```python
from build123d import *

# Parameters (mm, degrees)
BOSS_EXTRUDE1_DEPTH    = 558.8
SKETCH2_W              = 1233.22752028
SKETCH2_H              = 1270
SKETCH2_W_2            = 864.480609306
SKETCH2_H_2            = 355.6
CUT_EXTRUDE1_DEPTH     = 756.196292364
FILLET1_R              = 213.36
FILLET2_R              = 76.2
FILLET5_R              = 106.68
SHELL1_T               = 19.05
SKETCH7_W              = 20.32
SKETCH7_H              = 152.4
SKETCH7_2_W            = 20.32
SKETCH7_2_H            = 152.4
CUT_EXTRUDE2_DEPTH     = 152.4
FILLET6_R              = 25.4
LPATTERN1_COUNT        = 3
LPATTERN1_PITCH        = 167.64
FILLET6_OF_LPATTERN1_R = 25.4
SKETCH10_R             = 12.7
CUT_EXTRUDE3_DEPTH     = 688.251792528


with BuildPart() as part:
    # Sketch1 → Boss-Extrude1 (new body)
    with BuildSketch(Plane(origin=(0, 0, 0), x_dir=(1, 0, 0), z_dir=(0, 1, 0))):
        Polygon((359.210244843, 0), (0, -359.210244843), (-359.210244843, 0), (0, 359.210244843), align=None)
    extrude(amount=BOSS_EXTRUDE1_DEPTH)

    # Sketch2 → Cut-Extrude1 (cut, through all)
    with BuildSketch(Plane(origin=(0, 558.8, 0), x_dir=(1, 0, 0), z_dir=(0, 1, 0))):
        with Locations((0, 127)):
            Rectangle(SKETCH2_W, SKETCH2_H)
        with Locations((0, 127)):
            Rectangle(SKETCH2_W_2, SKETCH2_H_2, mode=Mode.SUBTRACT)
    extrude(amount=-CUT_EXTRUDE1_DEPTH, mode=Mode.SUBTRACT)

    # Fillet1
    # the kernel refuses this fillet: 213.36 mm, written as the material it takes off along each edge
    with BuildSketch(Plane(origin=(359.210244843, -399.180090434, 0), x_dir=(-0.707106781186546, 0, 0.707106781186549), z_dir=(0, 1, 0))) as fillet1_piece_1:
        with BuildLine():
            CenterArc((213.36, -159.672036174), FILLET1_R, 131.550696865, 48.449303135)
            Line((0, -159.672036174), (-4.2672, -159.672036174))
            Line((-4.2672, -159.672036174), (-4.2672, 0))
            Line((-4.2672, 0), (0, 4.2672))
            ThreePointArc((0, 4.2672), (35.921024484, 4.2672), (69.011689948, 3.193440723))
            Line((69.011689948, 3.193440723), (71.842048969, 0))
        make_face()
    extrude(amount=1357.160180869, mode=Mode.SUBTRACT)
    with BuildSketch(Plane(origin=(-359.210244843, -399.180090434, 0), x_dir=(0.707106781186546, 0, -0.7071067811865489), z_dir=(0, 1, 0))) as fillet1_piece_2:
        with BuildLine():
            CenterArc((159.672036174, -213.36), FILLET1_R, 90, 48.449303135)
            Line((0, -71.842048969), (-3.193440723, -69.011689948))
            ThreePointArc((-3.193440723, -69.011689948), (-4.2672, -35.921024484), (-4.2672, 0))
            Line((-4.2672, 0), (0, 4.2672))
            Line((0, 4.2672), (159.672036174, 4.2672))
            Line((159.672036174, 4.2672), (159.672036174, 0))
        make_face()
    extrude(amount=1357.160180869, mode=Mode.SUBTRACT)

    # Fillet2
    fillet2_edges = [part.edges().sort_by_distance(p)[0] for p in [
        (54.410244843, 279.4, -304.8),
        (-54.410244843, 279.4, -304.8),
    ]]
    fillet(fillet2_edges, radius=FILLET2_R)

    # Fillet5
    fillet5_edges = [part.edges().sort_by_distance(p)[0] for p in [
        (308.410244843, 279.4, 50.8),
        (-308.410244843, 279.4, 50.8),
    ]]
    fillet(fillet5_edges, radius=FILLET5_R)

    # Shell1 (no face opened: a closed hollow body)
    add(offset(amount=-SHELL1_T, mode=Mode.PRIVATE), mode=Mode.SUBTRACT)

    # Cut-Sweep1: sweep along a path in Sketch8
    with BuildLine(Plane(origin=(0, 558.8, 0), x_dir=(1, 0, 0), z_dir=(0, 1, 0))) as cut_sweep1_path:
        Line((0, -50.8), (-152.461942009, -50.8))
        ThreePointArc((-152.461942009, -50.8), (-251.021410537, 15.055331435), (-227.896093426, 131.314151417))
        Line((-227.896093426, 131.314151417), (-139.3067744, 219.903470443))
    # Sketch7 → Cut-Sweep1 (sweep, cut)
    with BuildSketch(Plane(origin=(0, 0, 0), x_dir=(0, 0, -1), z_dir=(1, 0, 0))):
        with Locations((-40.64, 444.5)):
            Rectangle(SKETCH7_W, SKETCH7_H)
    cut_sweep1 = sweep(path=cut_sweep1_path.line, mode=Mode.SUBTRACT)

    # Sketch7<2> → Cut-Extrude2 (cut)
    with BuildSketch(Plane(origin=(0, 0, 0), x_dir=(0, 0, -1), z_dir=(1, 0, 0))):
        with Locations((-40.64, 444.5)):
            Rectangle(SKETCH7_2_W, SKETCH7_2_H)
    cut_extrude2 = extrude(amount=CUT_EXTRUDE2_DEPTH, mode=Mode.SUBTRACT)

    # Fillet6
    fillet6_edges = [part.edges().sort_by_distance(p)[0] for p in [
        (-132.571582309, 520.7, -213.168278352),
        (-132.571582309, 368.3, -213.168278352),
        (152.4, 368.3, 41.275),
        (152.4, 520.7, 41.275),
    ]]
    fillet(fillet6_edges, radius=FILLET6_R)

    # LPattern1: Cut-Sweep1, Cut-Extrude2 ×3
    with Locations(*[(0, -i * LPATTERN1_PITCH, 0) for i in range(1, LPATTERN1_COUNT)]):
        add(cut_sweep1, mode=Mode.SUBTRACT)
        add(cut_extrude2, mode=Mode.SUBTRACT)

    # Fillet6 of LPattern1
    fillet6_of_lpattern1_edges = [part.edges().sort_by_distance(p)[0] for p in [
        (-132.571582309, 353.06, -213.168278352),
        (-132.571582309, 200.66, -213.168278352),
        (152.4, 200.66, 41.275),
        (152.4, 353.06, 41.275),
        (-132.571582309, 185.42, -213.168278352),
        (-132.571582309, 33.02, -213.168278352),
        (152.4, 33.02, 41.275),
        (152.4, 185.42, 41.275),
    ]]
    fillet(fillet6_of_lpattern1_edges, radius=FILLET6_OF_LPATTERN1_R)

    # Sketch10 → Cut-Extrude3 (cut, through all)
    with BuildSketch(Plane(origin=(0, 558.8, 0), x_dir=(1, 0, 0), z_dir=(0, 1, 0))):
        with Locations(Location((152.461942009, 55.88, 0), (0, 0, 270))):
            Circle(SKETCH10_R)
    extrude(amount=-CUT_EXTRUDE3_DEPTH, mode=Mode.SUBTRACT)


solid = part.part
```
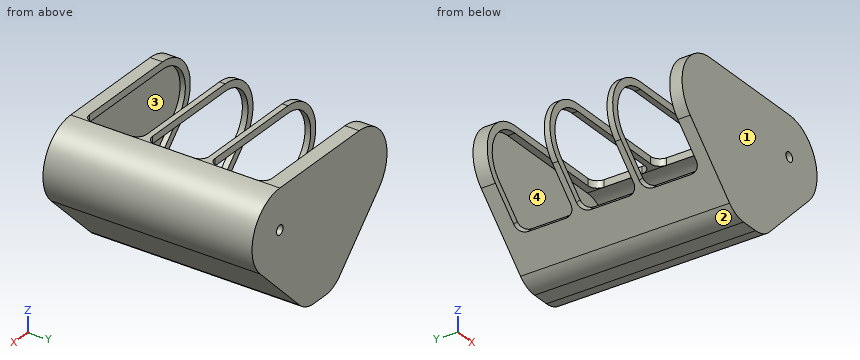
Design review of the part built by this model. Coordinates are the model's own, in mm. Face numbers are marked on the shaded views. Coordinates: 2 decimals unless noted, no trailing zeros. Loops run counter-clockwise (first coordinate to the right, second up) from the corner with the lowest first, then second, coordinate; pieces in that order, holes last.
Q1. We need section B-B on z = -261. State the section outline as (x, y) points, and give its area (3 significant figures).
Reported:
outline: (-98.21, 0) - (98.21, 0) - (98.21, 558.8) - (-98.21, 558.8) - close; hole (-71.27, 19.05) - (71.27, 19.05) - (71.27, 539.75) - (-71.27, 539.75) - close
area: 35,500 mm2
Q2. To check wall thickness, follow line 1 (Y direction, x = -173, z = 29.5); line 2 (X direction, y = 551.5, z = -55.88); line 3 (Y direction, x = 146, z = 14.5). State the ranges of each line that lie inside material, in increasing order.
Reported:
line 1: y = 0 to 33.02, 185.42 to 200.66, 353.06 to 368.3, 520.7 to 558.8
line 2: x = -259.14 to 139.76, 165.16 to 259.14
line 3: y = 0 to 19.05, 539.75 to 558.8
Q3. We need section A-A on x = 112. State the section outline as (y, z) points.
Reported:
outline: (0, -247.21) - (558.8, -247.21) - (558.8, 50.8) - (520.7, 50.8) - (520.7, 31.75) - (539.75, 31.75) - (539.75, -220.27) - (19.05, -220.27) - (19.05, 31.75) - (33.02, 31.75) - (33.02, 50.8) - (0, 50.8) - close; (185.42, 31.75) - (200.66, 31.75) - (200.66, 50.8) - (185.42, 50.8) - close; (353.06, 31.75) - (368.3, 31.75) - (368.3, 50.8) - (353.06, 50.8) - close
Q4. The part is to be moulded in two halves that separate along X. For the marked faces 1, 2, 3 and 4, say which applies: +X half, -X half, draft (parallel to the pull), parting line (faces both ways), or undercut.
Reported:
face 1: draft
face 2: -X half
face 3: undercut
face 4: undercut
Q5. We need section C-C on z = -51. State how many separate pieces and enclosed holes the cut face has, and give its area (3 significant figures).
Reported:
separate pieces: 5
enclosed holes: 0
area: 30,000 mm2
Q6. For pin 1 (12 mm diameter, centred on x = 126.5, z = -164, fed in from -Y); pin 2 (4 mm diameter, centred on y = 165.5, z = -121.5, fed in from -X); pin 3 (2 mm diameter, centred on y = 498.5, z = -31.5, fed in from +X); pin 4 (21 mm diameter, centred on y = 132.5, z = 42, fed in from -X), all flat-tipped, find the tip position at first contact; note any pin that passes through.
Reported:
pin 1: stops at y = 0
pin 2: stops at x = 208.77
pin 3: stops at x = 256.55
pin 4: stops at x = 152.4
